Verification items for the finished model (mm, model axes). Round coordinates to 2 decimals unless told otherwise and drop trailing zeros. Loops run counter-clockwise (first coordinate to the right, second up) from the corner with the lowest first, then second, coordinate; pieces in that order, holes last.
from build123d import *

# Parameters (mm, degrees)
SCHIZZO1_R                   = 139
SCHIZZO1_R_2                 = 103.5
ESTRUSIONE_ESTRUSIONE1_DEPTH = 2.5


with BuildPart() as part:
    # Schizzo1 → Estrusione-Estrusione1 (new, symmetric)
    with BuildSketch(Plane(origin=(0, 0, 0), x_dir=(1, 0, 0), z_dir=(0, 1, 0))):
        with Locations(Location((0, 0, 0), (0, 0, 270))):
            Circle(SCHIZZO1_R)
        with Locations(Location((0, 0, 0), (0, 0, 270))):
            Circle(SCHIZZO1_R_2, mode=Mode.SUBTRACT)
        with BuildLine():
            ThreePointArc((-115.468480571, 24.098722638), (-120.890722726, 32.381191474), (-129.173191562, 26.958949319))
            ThreePointArc((-129.173191562, 26.958949319), (-131.956426015, 0), (-129.173191562, -26.958949319))
            ThreePointArc((-129.173191562, -26.958949319), (-120.890722726, -32.381191474), (-115.468480571, -24.098722638))
            ThreePointArc((-115.468480571, -24.098722638), (-117.956426015, 0), (-115.468480571, 24.098722638))
        make_face(mode=Mode.SUBTRACT)
        with BuildLine():
            ThreePointArc((-24.098722638, 115.468480571), (-32.381191474, 120.890722726), (-26.958949319, 129.173191562))
            ThreePointArc((-26.958949319, 129.173191562), (0, 131.956426015), (26.958949319, 129.173191562))
            ThreePointArc((26.958949319, 129.173191562), (32.381191474, 120.890722726), (24.098722638, 115.468480571))
            ThreePointArc((24.098722638, 115.468480571), (0, 117.956426015), (-24.098722638, 115.468480571))
        make_face(mode=Mode.SUBTRACT)
        with BuildLine():
            ThreePointArc((115.468480571, 24.098722638), (120.890722726, 32.381191474), (129.173191562, 26.958949319))
            ThreePointArc((129.173191562, 26.958949319), (131.956426015, 0), (129.173191562, -26.958949319))
            ThreePointArc((129.173191562, -26.958949319), (120.890722726, -32.381191474), (115.468480571, -24.098722638))
            ThreePointArc((115.468480571, -24.098722638), (117.956426015, 0), (115.468480571, 24.098722638))
        make_face(mode=Mode.SUBTRACT)
        with BuildLine():
            ThreePointArc((24.098722638, -115.468480571), (32.381191474, -120.890722726), (26.958949319, -129.173191562))
            ThreePointArc((26.958949319, -129.173191562), (0, -131.956426015), (-26.958949319, -129.173191562))
            ThreePointArc((-26.958949319, -129.173191562), (-32.381191474, -120.890722726), (-24.098722638, -115.468480571))
            ThreePointArc((-24.098722638, -115.468480571), (0, -117.956426015), (24.098722638, -115.468480571))
        make_face(mode=Mode.SUBTRACT)
    extrude(amount=ESTRUSIONE_ESTRUSIONE1_DEPTH, both=True)


solid = part.part
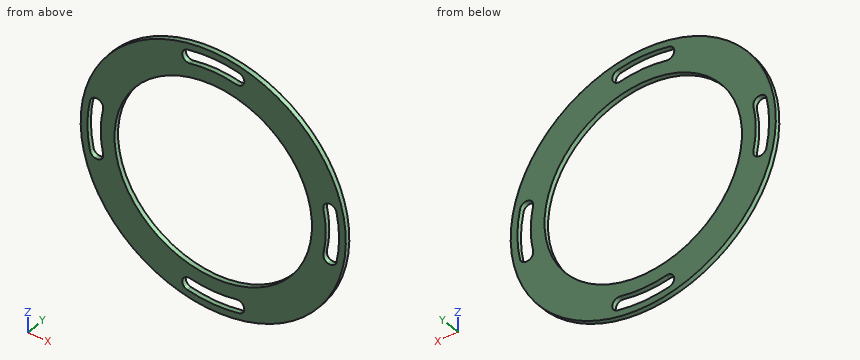
1. Section check D-D (z = 62). Enter the section's corners in (x, y), then the cut area to 3 significant figures.
2. Gauge pin test, flat ends, axial feed: P1, Ø8, axis at x = -63.5, z = -79, coming from the +Y side; P2, Ø2, axis at x = -39, y = -1, coming from the -Z side; P3, Ø2, axis at x = 85, y = 0, coming from the -Z side. Record the tip position at first contact, or that the pin passes through.
3. Section check B-B (z = 0). Enter the section's corners in (x, y), then the cut area to 3 significant figures.
4. Section check C-C (x = 0). Enter the section's corners in (y, z).
5. Scan lines: L1, parallel to X at y = 1.2, z = 0; L2, parallel to Z at x = 17.5, y = -0.2; L3, parallel to Z at x = 23, y = -0.75. Record each from-to range of solid material in increasing order.
6. Section check A-A (y = 0.45). Enter the section's corners in (x, z), then the cut area to 4 significant figures.
Taken from the geometry:
1. outline: (-124.41, -2.5) - (-82.87, -2.5) - (-82.87, 2.5) - (-124.41, 2.5) - close; (82.87, -2.5) - (124.41, -2.5) - (124.41, 2.5) - (82.87, 2.5) - close
1. area: 415 mm2
2. P1: stops at y = 2.5
2. P2: stops at z = -133.7
2. P3: stops at z = -110.75
3. outline: (-139, -2.5) - (-131.96, -2.5) - (-131.96, 2.5) - (-139, 2.5) - close; (-117.96, -2.5) - (-103.5, -2.5) - (-103.5, 2.5) - (-117.96, 2.5) - close; (103.5, -2.5) - (117.96, -2.5) - (117.96, 2.5) - (103.5, 2.5) - close; (131.96, -2.5) - (139, -2.5) - (139, 2.5) - (131.96, 2.5) - close
3. area: 215 mm2
4. outline: (-2.5, -139) - (2.5, -139) - (2.5, -131.96) - (-2.5, -131.96) - close; (-2.5, -117.96) - (2.5, -117.96) - (2.5, -103.5) - (-2.5, -103.5) - close; (-2.5, 103.5) - (2.5, 103.5) - (2.5, 117.96) - (-2.5, 117.96) - close; (-2.5, 131.96) - (2.5, 131.96) - (2.5, 139) - (-2.5, 139) - close
5. L1: x = -139 to -131.96, -117.96 to -103.5, 103.5 to 117.96, 131.96 to 139
5. L2: z = -137.89 to -130.79, -116.65 to -102.01, 102.01 to 116.65, 130.79 to 137.89
5. L3: z = -137.08 to -129.94, -115.69 to -100.91, 100.91 to 115.69, 129.94 to 137.08
6. outline: circle Ø278 at (0, 0); hole (-129.17, -26.96) arc R7 ccw to (-115.47, -24.1) arc R117.96 cw to (-115.47, 24.1) arc R7 ccw to (-129.17, 26.96) arc R131.96 ccw to start; hole circle Ø207 at (0, 0); hole (-26.96, -129.17) arc R131.96 ccw to (26.96, -129.17) arc R7 ccw to (24.1, -115.47) arc R117.96 cw to (-24.1, -115.47) arc R7 ccw to start; hole (-26.96, 129.17) arc R7 ccw to (-24.1, 115.47) arc R117.96 cw to (24.1, 115.47) arc R7 ccw to (26.96, 129.17) arc R131.96 ccw to start; hole (115.47, -24.1) arc R7 ccw to (129.17, -26.96) arc R131.96 ccw to (129.17, 26.96) arc R7 ccw to (115.47, 24.1) arc R117.96 cw to start
6. area: 23,550 mm2
